The listing builds one solid part. Answer for the finished solid, in the listing's coordinates (mm). A direction names the side the tool comes from. Coordinates: 2 decimals unless noted, no trailing zeros. Write each loop counter-clockwise with the first axis right and the second up, starting at its lowest first coordinate (ties: lowest second). Pieces come first, ordered by that corner, then holes.
from build123d import *

# Parameters (mm, degrees)
SKETCH1_R                     = 13.843
SKETCH1_R_2                   = 11.303
BOSS_EXTRUDE1_DEPTH           = 7.62
BOSS_EXTRUDE4_DEPTH           = 1.5
BOSS_EXTRUDE4_DEPTH_BACK      = 7.62
SKETCH6_R                     = 17.78
SKETCH6_R_2                   = 16.51
BOSS_EXTRUDE5_DEPTH           = 9.12
BOSS_EXTRUDE6_START           = -2.54
BOSS_EXTRUDE6_OUTLINE_W       = 47.683186112
BOSS_EXTRUDE6_OUTLINE_H       = 47.683186112
BOSS_EXTRUDE6_OUTLINE_R       = 0.801080814
BOSS_EXTRUDE6_OUTLINE_R_2     = 13.843
BOSS_EXTRUDE6_DEPTH           = 2.54
SKETCH11_W                    = 2.4
SKETCH11_H                    = 2.54
M4_CLEARANCE_HOLE2_AT_2_COUNT = 2
M4_CLEARANCE_HOLE2_AT_2_PITCH = 35.921024484
M4_CLEARANCE_HOLE2_AT_3_COUNT = 2
M4_CLEARANCE_HOLE2_AT_3_PITCH = 50.8
M4_CLEARANCE_HOLE2_AT_4_COUNT = 2
M4_CLEARANCE_HOLE2_AT_4_PITCH = 35.921024484
FILLET1_R                     = 2.54
BOSS_EXTRUDE7_START           = 5.08
SKETCH12_R                    = 16.51
SKETCH12_R_2                  = 13.843
BOSS_EXTRUDE7_DEPTH           = 5.08
SKETCH8_R                     = 2.625
CUT_EXTRUDE2_DEPTH            = 41.597607221
FILLET2_R                     = 2.54


# Read off the part's stored shape, not the designer's step: Boss-Extrude6
with BuildPart() as part:
    # Sketch1 → Boss-Extrude1 (new body)
    with BuildSketch(Plane(origin=(0, 0, 0), x_dir=(1, 0, 0), z_dir=(0, 1, 0))):
        with Locations(Location((0, 0, 0), (0, 0, 90))):
            Circle(SKETCH1_R)
        with Locations(Location((0, 0, 0), (0, 0, 90))):
            Circle(SKETCH1_R_2, mode=Mode.SUBTRACT)
    extrude(amount=BOSS_EXTRUDE1_DEPTH)

    # Boss-Extrude6 outline → Boss-Extrude6 (add)
    with BuildSketch(Plane(origin=(0, 7.62, 0), x_dir=(1, 0, 0), z_dir=(0, 1, 0)).offset(BOSS_EXTRUDE6_START)):
        Rectangle(BOSS_EXTRUDE6_OUTLINE_W, BOSS_EXTRUDE6_OUTLINE_H)
        with Locations((-17.960512242, -17.960512242)):
            Circle(BOSS_EXTRUDE6_OUTLINE_R, mode=Mode.SUBTRACT)
        with Locations((17.960512242, -17.960512242)):
            Circle(BOSS_EXTRUDE6_OUTLINE_R, mode=Mode.SUBTRACT)
        with Locations((-17.960512242, 17.960512242)):
            Circle(BOSS_EXTRUDE6_OUTLINE_R, mode=Mode.SUBTRACT)
        Circle(BOSS_EXTRUDE6_OUTLINE_R_2, mode=Mode.SUBTRACT)
        with Locations((17.960512242, 17.960512242)):
            Circle(BOSS_EXTRUDE6_OUTLINE_R, mode=Mode.SUBTRACT)
    extrude(amount=BOSS_EXTRUDE6_DEPTH)

    # Sketch11 → M4 Clearance Hole2 (revolve, cut)
    with BuildSketch(Plane(origin=(17.960512242, 5.08, -17.960512242), x_dir=(0, 0, -1), z_dir=(1, 0, 0))):
        with Locations((1.2, 1.27)):
            Rectangle(SKETCH11_W, SKETCH11_H)
    m4_clearance_hole2 = revolve(axis=Axis((17.960512242, -1.27, -17.960512242), (0, 1, 0)), mode=Mode.SUBTRACT)

    # M4 Clearance Hole2 at 2: M4 Clearance Hole2 ×2
    with Locations(*[(-i * M4_CLEARANCE_HOLE2_AT_2_PITCH, 0, 0) for i in range(1, M4_CLEARANCE_HOLE2_AT_2_COUNT)]):
        add(m4_clearance_hole2, mode=Mode.SUBTRACT)

    # M4 Clearance Hole2 at 3: M4 Clearance Hole2 ×2
    with Locations(*[Vector(-0.7071067811865477, 0, 0.7071067811865475) * (i * M4_CLEARANCE_HOLE2_AT_3_PITCH) for i in range(1, M4_CLEARANCE_HOLE2_AT_3_COUNT)]):
        add(m4_clearance_hole2, mode=Mode.SUBTRACT)

    # M4 Clearance Hole2 at 4: M4 Clearance Hole2 ×2
    with Locations(*[(0, 0, i * M4_CLEARANCE_HOLE2_AT_4_PITCH) for i in range(1, M4_CLEARANCE_HOLE2_AT_4_COUNT)]):
        add(m4_clearance_hole2, mode=Mode.SUBTRACT)

    # Fillet1
    fillet1_edges = [part.edges().sort_by_distance(p)[0] for p in [
        (23.841593056, 6.35, -23.841593056),
        (23.841593056, 6.35, 23.841593056),
        (-23.841593056, 6.35, 23.841593056),
        (-23.841593056, 6.35, -23.841593056),
    ]]
    fillet(fillet1_edges, radius=FILLET1_R)



with BuildPart() as body_2:
    # Sketch6 → Boss-Extrude4 (new, two sides: drawn at the far end of the back side and taken through both)
    with BuildSketch(Plane.XZ.offset(-BOSS_EXTRUDE4_DEPTH_BACK)):
        with Locations(Location((0, 0, 0), (0, 0, 90))):
            Circle(SKETCH6_R)
        with Locations(Location((0, 0, 0), (0, 0, 90))):
            Circle(SKETCH6_R_2, mode=Mode.SUBTRACT)
    extrude(amount=BOSS_EXTRUDE4_DEPTH + BOSS_EXTRUDE4_DEPTH_BACK)

    # Sketch7 → Boss-Extrude5 (add)
    with BuildSketch(Plane.XZ.offset(1.5)):
        Polygon((-18.868493037, 6.35), (-31.568493037, 6.35), (-31.568493037, -6.35), (-18.868493037, -6.35), (-16.578258023, -6.35), (-16.578258023, 6.35), align=None)
        Polygon((18.868493037, 6.35), (16.578258023, 6.35), (16.578258023, -6.35), (18.868493037, -6.35), (31.568493037, -6.35), (31.568493037, 6.35), align=None)
    extrude(amount=-BOSS_EXTRUDE5_DEPTH)


with BuildPart() as part_1:
    add(part.part)

    add(body_2.part)  # Boss-Extrude7 merges body 2
    # Sketch12 → Boss-Extrude7 (add)
    with BuildSketch(Plane.XZ.offset(-5.08).offset(BOSS_EXTRUDE7_START)):
        with Locations(Location((0, 0, 0), (0, 0, 90))):
            Circle(SKETCH12_R)
        Circle(SKETCH12_R_2, mode=Mode.SUBTRACT)
    extrude(amount=-BOSS_EXTRUDE7_DEPTH)

    # Sketch8 → Cut-Extrude2 (cut, through all)
    with BuildSketch(Plane.XZ.offset(1.5)):
        with Locations(Location((-24.087949006, 0, 0), (0, 0, 270))):
            Circle(SKETCH8_R)
        with Locations(Location((24.087949006, 0, 0), (0, 0, 90))):
            Circle(SKETCH8_R)
    extrude(amount=-CUT_EXTRUDE2_DEPTH, mode=Mode.SUBTRACT)

    # Fillet2
    fillet2_edges = [part_1.edges().sort_by_distance(p)[0] for p in [
        (-31.568493037, 3.06, 6.35),
        (-31.568493037, 3.06, -6.35),
        (-16.607404975, 1.79, -6.35),
        (31.568493037, 3.06, -6.35),
        (16.607404975, 1.79, 6.35),
        (31.568493037, 3.06, 6.35),
        (16.607404975, 1.79, -6.35),
        (23.841593056, 6.35, -6.35),
        (-23.841593056, 6.35, -6.35),
        (-16.607404975, 1.79, 6.35),
        (-23.841593056, 6.35, 6.35),
        (23.841593056, 6.35, 6.35),
    ]]
    fillet(fillet2_edges, radius=FILLET2_R)


solid = part_1.part
Q1. Determine the mould class of faces 1 (the face through (0, 6, 23.842)), 2 (the face through (31.568, 3, 0)), 3 (the face through (10.028, 3.757, -5.216)) for opening direction Z: released by +Z, released by -Z, zero draft, split by the parting line, or undercut.
Answers below:
face 1: released by +Z
face 2: zero draft
face 3: undercut
Q2. The part is cut by section C-C, the plane z = 5. Write down the section's boundary in (x, y), then the cut area to 3 significant figures.
Answers below:
outline: (-31.27, -1.5) - (-15.73, -1.5) - (-15.73, 0) - (-10.14, 0) - (-10.14, 7.62) - (-31.27, 7.62) - close; (10.14, 0) - (15.73, 0) - (15.73, -1.5) - (31.27, -1.5) - (31.27, 7.62) - (10.14, 7.62) - close
area: 369 mm2
Q3. Which of the six approach directions +Z, -Z, +X, -X, +Y, -Y give full straight-line access (tool end or side, diameter ignored) to faces 4 (the face through (10.05, -0.74, -13.1)), 5 (the face through (16.908, 1.836, 6.747)), 6 (the face through (-16.942, 1.836, 6.726)), 7 (the face through (0, 5.08, 19)), 8 (the face through (-17.041, 6.368, -20.178))?
Answers below:
face 4: -Y
face 5: +Z, +X, -Y
face 6: +Z, -X, -Y
face 7: +Z, -Y
face 8: +Y, -Y
Q4. Given pin 1 (3 mm diameter, centred on y = 6.5, z = 15.5, fed in from +X); pin 2 (2 mm diameter, centred on y = 0, z = 15.5, fed in from -X); pin 3 (0.8 mm diameter, centred on y = 6.5, z = 14, fed in from -X); pin 4 (3 mm diameter, centred on x = -17.96, z = -17.96, fed in from -Y), each flat-ended and moving along its own axis, determine where each tip first touches the part or whether it passes through.
Answers below:
pin 1: stops at x = 23.84
pin 2: stops at x = -10.29
pin 3: stops at x = -23.84
pin 4: passes through
Q5. The part is cut by section A-A, the plane x = 0. Write down the section's boundary in (y, z), then the cut area to 3 significant figures.
Answers below:
outline: (-1.5, -17.78) - (5.08, -17.78) - (5.08, -23.84) - (7.62, -23.84) - (7.62, -11.3) - (0, -11.3) - (0, -16.51) - (-1.5, -16.51) - close; (-1.5, 16.51) - (0, 16.51) - (0, 11.3) - (7.62, 11.3) - (7.62, 23.84) - (5.08, 23.84) - (5.08, 17.78) - (-1.5, 17.78) - close
area: 133 mm2
Q6. The part is cut by section B-B, the plane z = 0. Write down the section's boundary in (x, y), then the cut area to 3 significant figures.
Answers below:
outline: (-31.57, -1.5) - (-26.71, -1.5) - (-26.71, 7.62) - (-31.57, 7.62) - close; (-21.46, -1.5) - (-16.51, -1.5) - (-16.51, 0) - (-11.3, 0) - (-11.3, 7.62) - (-21.46, 7.62) - close; (11.3, 0) - (16.51, 0) - (16.51, -1.5) - (21.46, -1.5) - (21.46, 7.62) - (11.3, 7.62) - close; (26.71, -1.5) - (31.57, -1.5) - (31.57, 7.62) - (26.71, 7.62) - close
area: 258 mm2
Q7. The part is cut by section D-D, the plane y = 6. State how many separate pieces and enclosed holes the cut face has, then the cut area to 3 significant figures.
Answers below:
separate pieces: 1
enclosed holes: 7
area: 1,950 mm2
Q8. Find the intervals of material crossed by probe 1 along X at (y, z) = (5, 0); probe 2 along X at (y, z) = (-0.35, 0); probe 3 along Y at (x, z) = (15.5, -20), in increasing order.
Answers below:
probe 1: x = -31.57 to -26.71, -21.46 to -11.3, 11.3 to 21.46, 26.71 to 31.57
probe 2: x = -31.57 to -26.71, -21.46 to -16.51, 16.51 to 21.46, 26.71 to 31.57
probe 3: y = 5.08 to 7.62
